```python
from build123d import *

# Parameters (mm, degrees)
SKETCH1_R           = 12.7
BOSS_EXTRUDE1_DEPTH = 2.54
SKETCH2_R           = 6.477
SKETCH2_R_2         = 6.223
CUT_EXTRUDE1_DEPTH  = 0.5
SKETCH3_R           = 3.302
SKETCH3_R_2         = 3.048
CUT_EXTRUDE2_DEPTH  = 0.5
SKETCH4_R           = 0.25
CUT_EXTRUDE3_DEPTH  = 0.5
SKETCH5_R           = 9.652
SKETCH5_R_2         = 9.398
CUT_EXTRUDE4_DEPTH  = 0.5
SKETCH6_W           = 25.165512812
SKETCH6_H           = 0.254
CUT_EXTRUDE5_DEPTH  = 0.5
SKETCH7_W           = 0.254
SKETCH7_H           = 25.09846579
CUT_EXTRUDE6_DEPTH  = 0.5
SKETCH8_R           = 6.477
CUT_EXTRUDE7_DEPTH  = 10


with BuildPart() as part:
    # Sketch1 → Boss-Extrude1 (new body)
    with BuildSketch(Plane(origin=(0, 0, 0), x_dir=(1, 0, 0), z_dir=(0, 1, 0))):
        with Locations(Location((0, 0, 0), (0, 0, 270))):
            Circle(SKETCH1_R)
    extrude(amount=BOSS_EXTRUDE1_DEPTH)

    # Sketch2 → Cut-Extrude1 (cut)
    with BuildSketch(Plane(origin=(0, 2.54, 0), x_dir=(1, 0, 0), z_dir=(0, 1, 0))):
        with Locations(Location((0, 0, 0), (0, 0, 270))):
            Circle(SKETCH2_R)
        with Locations(Location((0, 0, 0), (0, 0, 270))):
            Circle(SKETCH2_R_2, mode=Mode.SUBTRACT)
    extrude(amount=-CUT_EXTRUDE1_DEPTH, mode=Mode.SUBTRACT)

    # Sketch3 → Cut-Extrude2 (cut)
    with BuildSketch(Plane(origin=(0, 2.54, 0), x_dir=(1, 0, 0), z_dir=(0, 1, 0))):
        with Locations(Location((0, 0, 0), (0, 0, 270))):
            Circle(SKETCH3_R)
        with Locations(Location((0, 0, 0), (0, 0, 270))):
            Circle(SKETCH3_R_2, mode=Mode.SUBTRACT)
    extrude(amount=-CUT_EXTRUDE2_DEPTH, mode=Mode.SUBTRACT)

    # Sketch4 → Cut-Extrude3 (cut)
    with BuildSketch(Plane(origin=(0, 2.54, 0), x_dir=(1, 0, 0), z_dir=(0, 1, 0))):
        with Locations(Location((0, 0, 0), (0, 0, 270))):
            Circle(SKETCH4_R)
    extrude(amount=-CUT_EXTRUDE3_DEPTH, mode=Mode.SUBTRACT)

    # Sketch5 → Cut-Extrude4 (cut)
    with BuildSketch(Plane(origin=(0, 2.54, 0), x_dir=(1, 0, 0), z_dir=(0, 1, 0))):
        with Locations(Location((0, 0, 0), (0, 0, 270))):
            Circle(SKETCH5_R)
        with Locations(Location((0, 0, 0), (0, 0, 270))):
            Circle(SKETCH5_R_2, mode=Mode.SUBTRACT)
    extrude(amount=-CUT_EXTRUDE4_DEPTH, mode=Mode.SUBTRACT)

    # Sketch6 → Cut-Extrude5 (cut)
    with BuildSketch(Plane(origin=(0, 2.54, 0), x_dir=(1, 0, 0), z_dir=(0, 1, 0))):
        Rectangle(SKETCH6_W, SKETCH6_H)
    extrude(amount=-CUT_EXTRUDE5_DEPTH, mode=Mode.SUBTRACT)

    # Sketch7 → Cut-Extrude6 (cut)
    with BuildSketch(Plane(origin=(0, 2.54, 0), x_dir=(1, 0, 0), z_dir=(0, 1, 0))):
        Rectangle(SKETCH7_W, SKETCH7_H)
    extrude(amount=-CUT_EXTRUDE6_DEPTH, mode=Mode.SUBTRACT)

    # Sketch8 → Cut-Extrude7 (cut)
    with BuildSketch(Plane(origin=(0, 2.54, 0), x_dir=(1, 0, 0), z_dir=(0, 1, 0))):
        with Locations(Location((0, 0, 0), (0, 0, 270))):
            Circle(SKETCH8_R)
    extrude(amount=-CUT_EXTRUDE7_DEPTH, mode=Mode.SUBTRACT)


solid = part.part
```
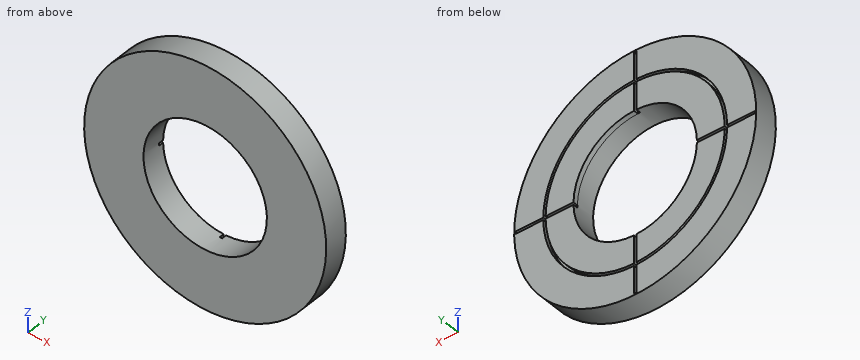
Design review of the part built by this model. Coordinates are the model's own, in mm. Give positions to 0.01 mm unless a question says otherwise; leave off trailing zeros. Write each loop counter-clockwise with the first axis right and the second up, starting at its lowest first coordinate (ties: lowest second). Pieces come first, ordered by that corner, then holes.
(1) Clearance check with flat-ended pins moving along their axes: pin 1 Ø1.5 at (y, z) = (1.5, 2) entering from -X; pin 2 Ø0.6 at (x, y) = (-7.5, 2.5) entering from +Z; pin 3 Ø0.6 at (y, z) = (2, -11.5) entering from -X. State where each tip first meets the part, or that it passes through.
Checked values:
pin 1: stops at x = -12.64
pin 2: stops at z = 10.46
pin 3: stops at x = -5.99
(2) Add section B-B (x = 1.75). Give the boundary of the cut face in (y, z).
Checked values:
outline: (0, -12.58) - (2.54, -12.58) - (2.54, -9.49) - (2.04, -9.49) - (2.04, -9.23) - (2.54, -9.23) - (2.54, -6.24) - (0, -6.24) - close; (0, 6.24) - (2.54, 6.24) - (2.54, 9.23) - (2.04, 9.23) - (2.04, 9.49) - (2.54, 9.49) - (2.54, 12.58) - (0, 12.58) - close
(3) Add section D-D (z = 8). Give the boundary of the cut face in (x, y), and give its area (3 significant figures).
Checked values:
outline: (-9.86, 0) - (9.86, 0) - (9.86, 2.54) - (5.4, 2.54) - (5.4, 2.04) - (4.93, 2.04) - (4.93, 2.54) - (0.13, 2.54) - (0.13, 2.04) - (-0.13, 2.04) - (-0.13, 2.54) - (-4.93, 2.54) - (-4.93, 2.04) - (-5.4, 2.04) - (-5.4, 2.54) - (-9.86, 2.54) - close
area: 49.5 mm2
(4) Add section C-C (y = 0.9). Give the boundary of the cut face in (x, z), and give its area (3 significant figures).
Checked values:
outline: circle Ø25.4 at (0, 0); hole circle Ø12.95 at (0, 0)
area: 375 mm2
(5) Add section A-A (z = -5.25). Give the boundary of the cut face in (x, y).
Checked values:
outline: (-11.56, 0) - (-3.79, 0) - (-3.79, 2.54) - (-7.79, 2.54) - (-7.79, 2.04) - (-8.1, 2.04) - (-8.1, 2.54) - (-11.56, 2.54) - close; (3.79, 0) - (11.56, 0) - (11.56, 2.54) - (8.1, 2.54) - (8.1, 2.04) - (7.79, 2.04) - (7.79, 2.54) - (3.79, 2.54) - close
(6) Wall thickness on line 1 along X through (y, z) = (2.45, -0.25); line 2 along X through (y, z) = (2.3, 2.75); line 3 along X through (y, z) = (0.7, 0): over which ranges is each line inside the solid? List them lowest first.
Checked values:
line 1: x = -12.7 to -9.65, -9.39 to -6.47, 6.47 to 9.39, 9.65 to 12.7
line 2: x = -12.4 to -9.25, -8.99 to -5.86, 5.86 to 8.99, 9.25 to 12.4
line 3: x = -12.7 to -6.48, 6.48 to 12.7
